Geometry: final body of the model. Coordinates: model frame, mm. Face numbers are marked on the shaded views. Give positions to 0.01 mm unless a question says otherwise; leave off trailing zeros. Loops run counter-clockwise (first coordinate to the right, second up) from the corner with the lowest first, then second, coordinate; pieces in that order, holes last.
1. Section B-B, the plane x = 25. State how many separate pieces and enclosed holes the cut face has, then the cut area to 3 significant figures.
2. First-contact query: P1, Ø4, axis at x = 25, y = 12, coming from the +Z side; P2, Ø3, axis at x = 6.5, y = 12.5, coming from the +Z side. Flat tips, straight axial feed; report the tip coordinate or a pass-through.
3. Draft query along Y for the marked faces 1, 2 and 3. Return one class per face: +Y half, -Y half, draft (parallel to the pull), parting line (faces both ways), or undercut.
4. Section A-A, the plane y = 4. Output: boundary loops of the cut face in (x, z), then the cut area to 3 significant figures.
5. Material intervals for line 1 along Y through (x, z) = (25, 2.25); line 2 along X through (y, z) = (4, 1.9); line 3 along X through (y, z) = (5.25, 4.8), sorted ascending.
6. Section C-C, the plane z = 2.9. Output: boundary loops of the cut face in (x, y), then the cut area to 3 significant figures.
from build123d import *

# Parameters (mm, degrees)
SKETCH1_W                                            = 30
SKETCH1_H                                            = 16
BOSS_EXTRUDE1_DEPTH                                  = 5
CSK_FOR_M3_HEX_SOCKET_COUNTERSUNK_HEAD_S_D           = 3.6
CSK_FOR_M3_HEX_SOCKET_COUNTERSUNK_HEAD_S_CSINK_D     = 6.94
CSK_FOR_M3_HEX_SOCKET_COUNTERSUNK_HEAD_S_CSINK_ANGLE = 90
FILLET1_R                                            = 3
FILLET2_R                                            = 0.5


with BuildPart() as part:
    # Sketch1 → Boss-Extrude1 (new body)
    with BuildSketch(Plane.XY):
        with Locations((15, 8)):
            Rectangle(SKETCH1_W, SKETCH1_H)
    extrude(amount=BOSS_EXTRUDE1_DEPTH)

    # CSK for M3 Hex Socket Countersunk Head Screw1 (through all)
    with Locations(Plane.XY.offset(5)):
        with Locations((5, 12), (25, 12), (25, 4), (5, 4)):
            CounterSinkHole(CSK_FOR_M3_HEX_SOCKET_COUNTERSUNK_HEAD_S_D / 2, CSK_FOR_M3_HEX_SOCKET_COUNTERSUNK_HEAD_S_CSINK_D / 2, counter_sink_angle=CSK_FOR_M3_HEX_SOCKET_COUNTERSUNK_HEAD_S_CSINK_ANGLE)

    # Fillet1
    fillet1_edges = [part.edges().sort_by_distance(p)[0] for p in [
        (0, 16, 2.5),
        (30, 16, 2.5),
        (30, 0, 2.5),
        (0, 0, 2.5),
    ]]
    fillet(fillet1_edges, radius=FILLET1_R)

    # Fillet2
    fillet2_edges = [part.edges().sort_by_distance(p)[0] for p in [
        (30, 8, 0),
        (30, 8, 5),
        (0, 8, 0),
        (15, 16, 0),
        (15, 0, 0),
        (0.878679656, 15.121320344, 0),
        (0.878679656, 0.878679656, 0),
        (29.121320344, 15.121320344, 0),
        (29.121320344, 0.878679656, 0),
        (15, 0, 5),
        (0, 8, 5),
        (15, 16, 5),
        (0.878679656, 15.121320344, 5),
        (0.878679656, 0.878679656, 5),
        (29.121320344, 15.121320344, 5),
        (29.121320344, 0.878679656, 5),
    ]]
    fillet(fillet2_edges, radius=FILLET2_R)


solid = part.part
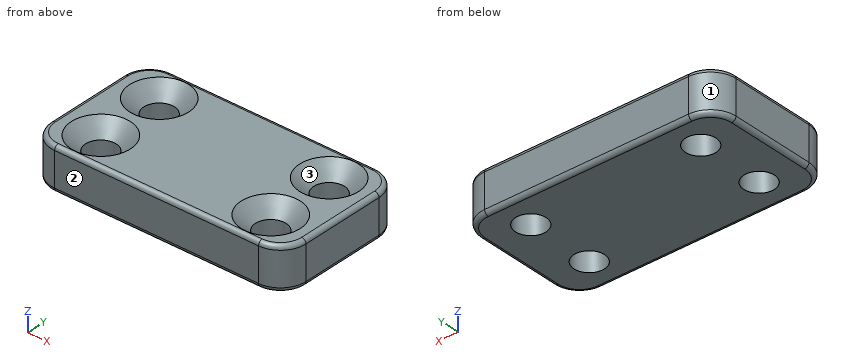
Answers below:
1. separate pieces: 3
1. enclosed holes: 0
1. area: 38.2 mm2
2. P1: stops at z = 3.53
2. P2: stops at z = 4.61
3. face 1: +Y half
3. face 2: -Y half
3. face 3: undercut
4. outline: (0, 0.5) arc R0.5 ccw to (0.5, 0) - (3.2, 0) - (3.2, 3.33) - (1.53, 5) - (0.5, 5) arc R0.5 ccw to (0, 4.5) - close; (6.8, 0) - (23.2, 0) - (23.2, 3.33) - (21.53, 5) - (8.47, 5) - (6.8, 3.33) - close; (26.8, 0) - (29.5, 0) arc R0.5 ccw to (30, 0.5) - (30, 4.5) arc R0.5 ccw to (29.5, 5) - (28.47, 5) - (26.8, 3.33) - close
4. area: 108 mm2
5. line 1: y = 0 to 2.2, 5.8 to 10.2, 13.8 to 16
5. line 2: x = 0 to 3.2, 6.8 to 23.2, 26.8 to 30
5. line 3: x = 0.1 to 1.98, 8.02 to 21.98, 28.02 to 29.9
6. outline: (0, 3) arc R3 ccw to (3, 0) - (27, 0) arc R3 ccw to (30, 3) - (30, 13) arc R3 ccw to (27, 16) - (3, 16) arc R3 ccw to (0, 13) - close; hole circle Ø3.6 at (5, 4); hole circle Ø3.6 at (5, 12); hole circle Ø3.6 at (25, 4); hole circle Ø3.6 at (25, 12)
6. area: 432 mm2
